```python
from build123d import *

# Parameters (mm, degrees)
F0_W     = 200
F0_H     = 200
F1_DEPTH = 2640
F2_W     = 200
F2_H     = 200
F2_W_2   = 120
F2_H_2   = 60
F3_DEPTH = 200


with BuildPart() as f1:
    # F0 (on Top) → F1 (new body)
    with BuildSketch(Plane.XY):
        with Locations((100, 100)):
            Rectangle(F0_W, F0_H)
    extrude(amount=F1_DEPTH)

    # F2 (on face) → F3 (cut)
    with BuildSketch(Plane.XY.offset(2640)):
        with Locations((100, 100)):
            Rectangle(F2_W, F2_H)
        with Locations((100, 100)):
            Rectangle(F2_W_2, F2_H_2, mode=Mode.SUBTRACT)
    extrude(amount=-F3_DEPTH, mode=Mode.SUBTRACT)


solid = f1.part
```
Design review of the part built by this model. Coordinates are the model's own, in mm. A direction names the side the tool comes from. Give positions to 0.01 mm unless a question says otherwise; leave off trailing zeros. Order: outer loops, then holes, each group sorted by start corner. A loop starts at its lowest first (then second) coordinate and runs counter-clockwise, first axis right, second up. Notation, with made-up numbers: (69.5, 54.5) -> (78.5, 54.5) arc R22 ccw to (78.5, 65.5) -> close; hole circle Ø8 at (62, 84). An arc over 180 degrees is marked (long way). Write item = value, one per line. Start each with the question number.
(1) For faces 4 (the face through (99, 70, 2541)), 5 (the face through (99, 130, 2541)), 6 (the face through (40, 100, 2541)), list the 3-axis set-ups (+Z, -Z, +X, -X, +Y, -Y) from which the entire face can be reached by the end or side of a thin tool; tool diameter is ignored.
(2) For pin 1 (10 mm diameter, centred on x = 42.5, y = 20.5, fed in from +Z); pin 2 (10 mm diameter, centred on y = 174.5, z = 731.5, fed in from -X), all flat-tipped, find the tip position at first contact; note any pin that passes through.
(3) To check wall thickness, follow line 1 along Y through (x, z) = (119.5, 2518); line 2 along Z through (x, y) = (69, 48). State the ranges of each line that lie inside material, in increasing order.
(4) We need section A-A on x = 108.5. Write out the cut boundary in (y, z), plus the area to 3 significant figures.
(5) We need section B-B on y = 106. Write out the cut boundary in (x, z).
(6) Mouldability with a two-part tool opening along Z and no side actions: class faces 1 (the face through (0, 99, 1203)), 2 (the face through (99, 100, 2640)), 3 (the face through (99, 101, 0)) as +Z half, -Z half, draft (parallel to the pull), parting line (faces both ways), or undercut.
Numbers:
q1.face_4 = +Z, +X, -X, -Y
q1.face_5 = +Z, +X, -X, +Y
q1.face_6 = +Z, -X, +Y, -Y
q2.pin_1 = 2440
q2.pin_2 = 0
q3.line_1 = 70 to 130
q3.line_2 = 0 to 2440
q4.outline = (0, 0) -> (200, 0) -> (200, 2440) -> (130, 2440) -> (130, 2640) -> (70, 2640) -> (70, 2440) -> (0, 2440) -> close
q4.area = 500,000 mm^2
q5.outline = (0, 0) -> (200, 0) -> (200, 2440) -> (160, 2440) -> (160, 2640) -> (40, 2640) -> (40, 2440) -> (0, 2440) -> close
q6.face_1 = draft
q6.face_2 = +Z half
q6.face_3 = -Z half
